Source: CAD feature listing. Evaluate the final solid. Frame: model axes, mm. A direction names the side the tool comes from. Give positions to 0.01 mm unless a question says otherwise; leave off trailing zeros. Loops run counter-clockwise (first coordinate to the right, second up) from the corner with the lowest first, then second, coordinate; pieces in that order, holes last.
Autodesk Inventor part; units mm, degrees
ref_plane "YZ Plane" through (0, 0, 0) normal (1, 0, 0) x (0, 1, 0)
ref_plane "XZ Plane" through (0, 0, 0) normal (0, 1, 0) x (-1, 0, 0)
ref_plane "XY Plane" through (0, 0, 0) normal (0, 0, 1) x (1, 0, 0)
sketch "Sketch1" plane through (0, 0, 0) normal (0, 0, 1) x (1, 0, 0)
  circle A0 centre (0, 0) radius 2.365
  dimension "d0" = 4.73
extrude "Extrusion1" add sketch "Sketch1" along normal blind 3
sketch "Sketch2" plane through (0, 0, 3) normal (0, 0, 1) x (1, 0, 0)
  circle A0 centre (0, 0) radius 2.94
  dimension "d3" = 5.88
extrude "Extrusion2" add sketch "Sketch2" along normal blind 5.9
thread "Thread1"
sketch "Sketch3" plane through (0, 0, 8.9) normal (0, 0, 1) x (1, 0, 0)
  circle A0 centre (0, 0) radius 2.94
  circle A1 centre (0, 0) radius 2.395
  dimension "d8" = 4.79
extrude "Extrusion3" add sketch "Sketch3" along normal blind 3.15 contours A1
sketch "Sketch4" plane through (0, 0, 12.05) normal (0, 0, 1) x (1, 0, 0)
  circle A0 centre (0, 0) radius 3.5
  dimension "d11" = 7
extrude "Extrusion4" add sketch "Sketch4" along normal blind 3.4
sketch "Sketch5" plane through (0, 0, 15.45) normal (0, 0, 1) x (1, 0, 0)
  line L0 (-1.8028, -3) -> (1.8028, -3)
  line L1 (9.1237, -3) -> (9.1237, 3)
  line L2 (1.8028, 3) -> (-1.8028, 3)
  line L3 (-9.1237, 3) -> (-9.1237, -3)
  line L4 (-9.1237, -3) -> (9.1237, 3) construction
  line L5 (9.1237, -3) -> (-9.1237, 3) construction
  circle A0 centre (0, 0) radius 3.5
  dimension "d14" = 6
extrude "Extrusion5" cut sketch "Sketch5" against normal blind 3.4 contours L0 A0 | A0 L2
sketch "Sketch6" plane through (0, 0, 15.45) normal (0, 0, 1) x (1, 0, 0)
  circle A0 centre (0, 0) radius 2.4
  dimension "d17" = 4.8
extrude "Extrusion6" add sketch "Sketch6" along normal blind 15.13
sketch "Sketch7" plane through (0, 0, 30.58) normal (0, 0, 1) x (1, 0, 0)
  circle A0 centre (0, 0) radius 2.965
  dimension "d20" = 5.93
extrude "Extrusion7" add sketch "Sketch7" along normal blind 25.17
thread "Thread2"
sketch "Sketch8" plane through (0, 0, 55.75) normal (0, 0, 1) x (1, 0, 0)
  circle A0 centre (0, 0) radius 1.2
  dimension "d25" = 2.4
extrude "Extrusion8" cut sketch "Sketch8" against normal through all
chamfer "Chamfer1" distance 1.5 angle 45 1 edges at (-1.2, 0, 55.75)
chamfer "Chamfer2" distance 0.5 angle 45 1 edges at (-1.2, 0, 0)
properties part number "feeder tube" material "Stainless Steel"
1) Ray query, probe 1 along X at (y, z) = (-0.1, 49); probe 2 along Y at (x, z) = (0, 23); probe 3 along Z at (x, y) = (2.5, 0.8). Return the intervals inside material, ascending.
Checks:
probe 1: x = -2.96 to -1.2, 1.2 to 2.96
probe 2: y = -2.4 to -1.2, 1.2 to 2.4
probe 3: z = 3 to 8.9, 12.05 to 15.45, 30.58 to 55.67
2) Cut plane D-D (z = 44.5). Return loops of the section in (x, y) (3 decimals), and give its area (3 significant figures).
Checks:
outline: circle Ø5.93 at (0, 0); hole circle Ø2.4 at (0, 0)
area: 23.1 mm2
3) Cut plane C-C (z = 14). Return loops of the section in (x, y).
Checks:
outline: (-1.8, -3) - (1.8, -3) arc R3.5 ccw to (1.8, 3) - (-1.8, 3) arc R3.5 ccw to start; hole circle Ø2.4 at (0, 0)
4) Reachability of faces 4 (the cylindrical face through (-0.643, 2.894, 42.989)), 5 (the flat face through (0, -3, 14)), 6 (the cylindrical face through (-0.519, 2.338, 10.453)), 7 (the cylindrical face through (2.8, -0.9, 5.9)) from +Z, -Z, +X, -X, +Y, -Y: full face, straight path, thin tool, end or side. Return the list, or none.
Checks:
face 4: +Z
face 5: +Z, -Z, +X, -X, -Y
face 6: none
face 7: -Z
5) Contact query for flat-ended pins moving along their axis: P1, Ø3, axis at x = 2, z = 48.5, coming from the -Y side; P2, Ø3, axis at y = -0.5, z = 38.5, coming from the -X side (3 decimals); P3, Ø3, axis at x = 0, y = 0, coming from the +Z side. Output: stop coordinate, or through.
Checks:
P1: stops at y = -2.92
P2: stops at x = -2.965
P3: stops at z = 54.55
6) Pull-direction query (X, two-part tool) for faces 1 (the flat face through (-2, -2, 12.05)), 2 (the cylindrical face through (-3.5, -0.1, 13.7)), 3 (the cylindrical face through (0.65, 1.01, 27.75)); classes: released by +X, released by -X, zero draft, split by the parting line, or undercut.
Checks:
face 1: zero draft
face 2: released by -X
face 3: undercut
